Job drawing, mm, ordinate dimensions from the low corner. One solid piece. A direction names the side the tool comes from. Give positions to 0.01 mm unless a question says otherwise; leave off trailing zeros. Write each loop counter-clockwise with the first axis right and the second up, starting at its lowest first coordinate (ties: lowest second). Pieces come first, ordered by that corner, then holes. Notation, with made-up numbers: (34.25, -32) - (93.25, -32) arc R26 cw to (93.25, -15) - close; hole circle Ø6 at (-7, 52). An arc over 180 degrees is marked (long way). Answer as a JSON object with one key per item and string values.
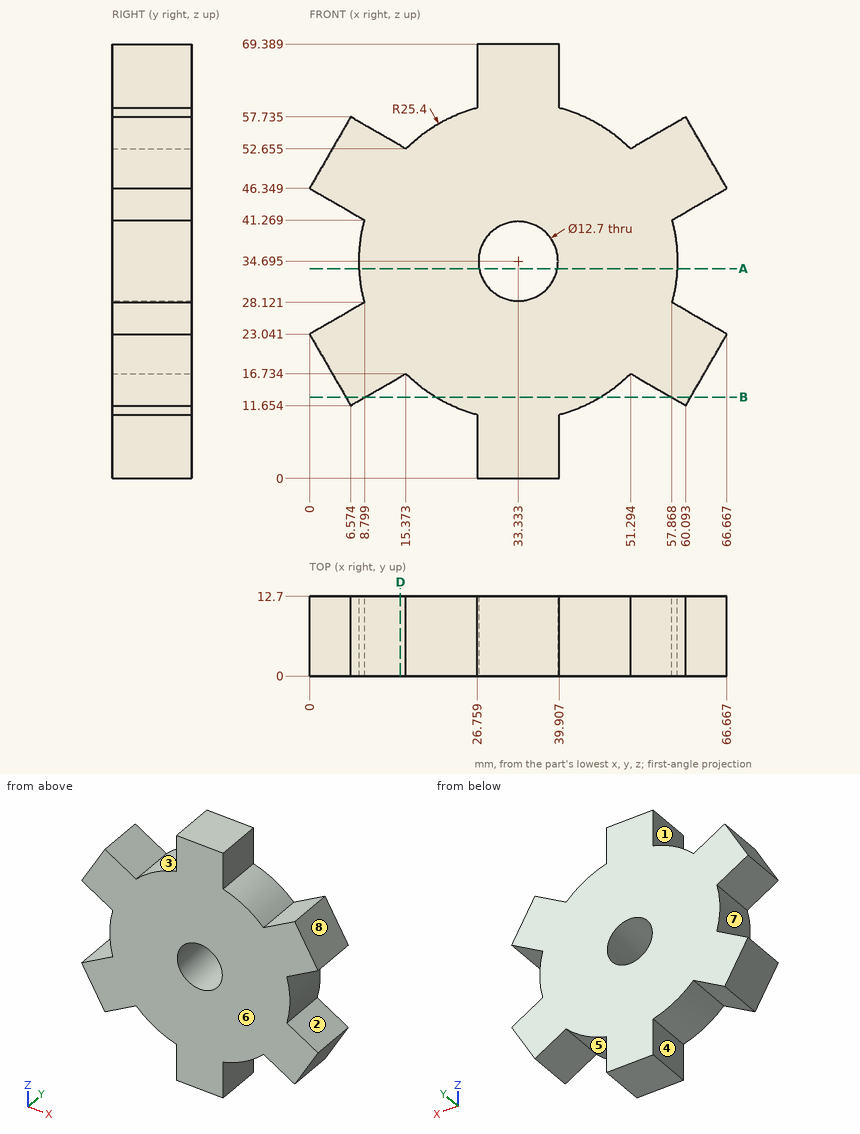
Item 1: Cut at A-A (z = 33.5). Give the cut face in (x, y) (1 decimal), and give its area (3 significant figures).
Entries:
{"outline": "(8, 0) - (27.1, 0) - (27.1, 12.7) - (8, 12.7) - close; (39.6, 0) - (58.7, 0) - (58.7, 12.7) - (39.6, 12.7) - close", "area": "486 mm2"}
Item 2: Probe line 1 (X direction, y = 6.25, z = 54.5) (1 decimal); line 2 (X direction, y = 9, z = 59.5); line 3 (Z direction, x = 60, y = 1.5). List the from-to ranges inside material, lowest first. Write a range as from..to.
Entries:
{"line 1": "4.7..12.2, 17.4..49.2, 54.5..62", "line 2": "26.76..39.91", "line 3": "11.71..26.89, 42.5..57.68"}
Item 3: Flat gauge pins, fed straight in: P1, Ø2, axis at x = 48, y = 4.5, coming from the +Z side (1 decimal); P2, Ø3, axis at y = 8.5, z = 44, coming from the +X side (1 decimal); P3, Ø5, axis at x = 12.5, y = 5, coming from the -Z side. Where does each tip first touch, or does it go through?
Entries:
{"P1": "z = 56.1", "P2": "x = 65.2", "P3": "z = 13.63"}
Item 4: Cut at D-D (x = 14.5). Give the cut face in (y, z).
Entries:
{"outline": "(0, 16.23) - (12.7, 16.23) - (12.7, 53.16) - (0, 53.16) - close"}
Item 5: Cut at B-B (z = 13). Give the cut face in (x, y) (1 decimal).
Entries:
{"outline": "(5.8, 0) - (8.9, 0) - (8.9, 12.7) - (5.8, 12.7) - close; (20.1, 0) - (46.5, 0) - (46.5, 12.7) - (20.1, 12.7) - close; (57.8, 0) - (60.9, 0) - (60.9, 12.7) - (57.8, 12.7) - close"}
Item 6: Which spindle directions (+Z, -Z, +X, -X, +Y, -Y) get a long thin tool onto all of the face, cutting with end or side? Do the marked faces 1, 2, 3, 4 and 5. Say none if no direction does.
Entries:
{"face 1": "+Z, -X, +Y, -Y", "face 2": "+X, +Y, -Y", "face 3": "+Z, +Y, -Y", "face 4": "-Z, -X, +Y, -Y", "face 5": "-Z, +Y, -Y"}
Item 7: Mould opens along Z. For the marked faces 6, 7 and 8 say: +Z half, -Z half, draft (parallel to the pull), parting line (faces both ways), or undercut.
Entries:
{"face 6": "draft", "face 7": "undercut", "face 8": "+Z half"}
